Autodesk Inventor part; units mm, degrees
ref_plane "YZ Plane" through (0, 0, 0) normal (1, 0, 0) x (0, 1, 0)
ref_plane "XZ Plane" through (0, 0, 0) normal (0, 1, 0) x (-1, 0, 0)
ref_plane "XY Plane" through (0, 0, 0) normal (0, 0, 1) x (1, 0, 0)
sketch "Sketch1" plane through (0, 0, 0) normal (0, 1, 0) x (-1, 0, 0)
  line L0 (0, 0) -> (-25.4, 0)
  line L1 (-25.4, 0) -> (-25.4, 25.4)
  line L2 (-25.4, 25.4) -> (0, 25.4)
  line L3 (0, 25.4) -> (0, 0)
  line L4 (-1.5875, 1.5875) -> (-23.8125, 1.5875)
  line L5 (-23.8125, 1.5875) -> (-23.8125, 23.8125)
  line L6 (-23.8125, 23.8125) -> (-1.5875, 23.8125)
  line L7 (-1.5875, 23.8125) -> (-1.5875, 1.5875)
  dimension "d0" = 25.4
  dimension "d2" = 25.4
  dimension "d3" = 1.5875
extrude "Extrusion1" add sketch "Sketch1" along normal blind 762
sketch "Sketch2" plane through (25.4, 0, 25.4) normal (1, 0, 0) x (0, 0, -1)
  line L0 (25.4, 0) -> (0, 0)
  line L1 (25.4, 0) -> (25.4, 762)
  line L2 (0, 762) -> (25.4, 762)
  line L3 (0, 0) -> (0, 762)
  line L4 (0, 0) -> (25.4, 3.783)
  line L5 (0, 603.4839) -> (25.4, 607.2669)
  dimension "d6" = 596.9
  dimension "d8" = 603.4839
extrude "Extrusion2" cut sketch "Sketch2" against normal blind 762 contours L0 L4 L1 | L3 L2 L1 L5
properties part number "Square Tube 5" material "Aluminum 6061"
Read the model definition and answer for the solid it produces. Units are mm, in the model's axes. A direction names the side the tool comes from. Coordinates: 2 decimals unless noted, no trailing zeros. Order: outer loops, then holes, each group sorted by start corner. A loop starts at its lowest first (then second) coordinate and runs counter-clockwise, first axis right, second up. Notation, with made-up numbers: (72, 68.5) - (130, 68.5) arc R12 ccw to (130, 75.5) - close; hole circle Ø11 at (85, 80.25). An arc over 180 degrees is marked (long way). Answer as a JSON object with one key per item and string values. Group by question number.
Item 1: Section B-B (x = 16) is taken. Give the vertices of the cut face in (y, z), plus the area to 3 significant figures.
Item 2: A tool of negligible diameter and unlimited length cuts with its end or side. For faces 1 (the face through (13, 301, 0)), 2 (the face through (13, 298, 23.812)), from which of +Z, -Z, +X, -X, +Y, -Y can it reach the whole face along a straight path? Write none if from no direction.
Item 3: Section C-C (z = 13) is taken. Give the vertices of the cut face in (x, y).
Item 4: The mould has two halves that part along Z. Classify faces 3 (the face through (24.048, 1.883, 12.759)), 4 (the face through (13, 301, 1.588)), 5 (the face through (13, 298, 25.4)): +Z half, -Z half, draft (parallel to the pull), parting line (faces both ways), or undercut.
Item 5: Section A-A (y = 284.5) is taken. Give the vertices of the cut face in (x, z).
Item 6: Consider probe 1 along X at (y, z) = (286, 10); probe 2 along Y at (x, z) = (19.5, 24.5). Determine where each line is inside the solid, lowest interval first. Write a range as from..to.
Results are:
{
 "1": {"outline": "(0, 25.4) - (0.24, 23.81) - (603.72, 23.81) - (603.48, 25.4) - close; (3.55, 1.59) - (3.78, 0) - (607.27, 0) - (607.03, 1.59) - close", "area": "1,920 mm^2"},
 "2": {"face 1": "-Z, +X, -X, +Y, -Y", "face 2": "+Y, -Y"},
 "3": {"outline": "(0, 1.85) - (1.59, 1.85) - (1.59, 605.33) - (0, 605.33) - close; (23.81, 1.85) - (25.4, 1.85) - (25.4, 605.33) - (23.81, 605.33) - close"},
 "4": {"face 3": "-Z half", "face 4": "undercut", "face 5": "+Z half"},
 "5": {"outline": "(0, 0) - (25.4, 0) - (25.4, 25.4) - (0, 25.4) - close; hole (1.59, 1.59) - (23.81, 1.59) - (23.81, 23.81) - (1.59, 23.81) - close"},
 "6": {"probe 1": "x = 0..1.59, 23.81..25.4", "probe 2": "y = 0.13..603.62"}
}
